from build123d import *

# Parameters (mm, degrees)
SKETCH1_W           = 12
SKETCH1_H           = 75
SKETCH1_W_2         = 50
SKETCH1_H_2         = 12
BOSS_EXTRUDE1_DEPTH = 12


with BuildPart() as part:
    # Sketch1 → Boss-Extrude1 (new body)
    with BuildSketch(Plane(origin=(0, 0, 0), x_dir=(1, 0, 0), z_dir=(0, 1, 0))):
        with Locations((-6, 75)):
            Rectangle(SKETCH1_W, SKETCH1_H)
        Polygon((0, 37.5), (0, 0), (25, 0), (25, 12), (75, 12), (75, 0), (100, 0), (0, 150), (0, 112.5), (12, 112.5), (12, 37.5), align=None)
        with Locations((50, -6)):
            Rectangle(SKETCH1_W_2, SKETCH1_H_2)
        with Locations((50, 6)):
            Rectangle(SKETCH1_W_2, SKETCH1_H_2)
        with Locations((6, 75)):
            Rectangle(SKETCH1_W, SKETCH1_H)
    extrude(amount=BOSS_EXTRUDE1_DEPTH)


solid = part.part
Geometry check sheet. Reference: the model listing, model coordinates, mm. A direction names the side the tool comes from. Give positions to 0.01 mm unless a question says otherwise; leave off trailing zeros. Loops run counter-clockwise (first coordinate to the right, second up) from the corner with the lowest first, then second, coordinate; pieces in that order, holes last. Notation, with made-up numbers: (64.25, 45) -> (100.25, 45) arc R22 cw to (100.25, 82) -> close; hole circle Ø8 at (-35.5, 77.5). An arc over 180 degrees is marked (long way). Answer in a Markdown table with one row per item. Add a question column.
1) Set-up check for faces 1 (the face through (25, 6, 6)), 2 (the face through (50.7, 5.92, -73.95)), 3 (the face through (-12, 6, -74)), 4 (the face through (75, 6, 6)), 5 (the face through (0, 6, -132)): record each of +Z, -Z, +X, -X, +Y, -Y from which the full face is reachable in a straight line by a thin tool's end or side.
2) Cross-section at B-B on z = -130.5. Record the boundary of the cut face in (x, y).
3) Cross-section at C-C on x = 9.5. Record the boundary of the cut face in (y, z), and give its area (3 significant figures).
4) Cross-section at A-A on y = 9.5. Record the boundary of the cut face in (x, z), and give its area (3 significant figures).
5) Material ranges on probe 1 along X at (y, z) = (6.5, -21.5); probe 2 along Z at (x, y) = (24, 1.75); probe 3 along Z at (x, y) = (30, 5.75), recorded low to high. Write a range as from..to.
6) Gauge pin test, flat ends, axial feed: P1, Ø3.5, axis at y = 8, z = -24, coming from the -X side; P2, Ø3, axis at x = 68.5, y = 9.5, coming from the -Z side; P3, Ø6, axis at x = -8, y = 7.5, coming from the +Z side. Record the tip position at first contact, or that the pin passes through.
Outcome:
| question | item | result |
|---|---|---|
| 1 | face 1 | +Z, -X, +Y, -Y |
| 1 | face 2 | -Z, +X, +Y, -Y |
| 1 | face 3 | +Z, -Z, -X, +Y, -Y |
| 1 | face 4 | +Z, +X, +Y, -Y |
| 1 | face 5 | -Z, -X, +Y, -Y |
| 2 | outline | (0, 0) -> (13, 0) -> (13, 12) -> (0, 12) -> close |
| 3 | outline | (0, -135.75) -> (12, -135.75) -> (12, 0) -> (0, 0) -> close |
| 3 | area | 1,630 mm^2 |
| 4 | outline | (-12, -112.5) -> (0, -112.5) -> (0, -150) -> (100, 0) -> (75, 0) -> (75, 12) -> (25, 12) -> (25, 0) -> (0, 0) -> (0, -37.5) -> (-12, -37.5) -> close |
| 4 | area | 9,000 mm^2 |
| 5 | probe 1 | x = 0..85.67 |
| 5 | probe 2 | z = -114..0 |
| 5 | probe 3 | z = -105..12 |
| 6 | P1 | stops at x = 0 |
| 6 | P2 | stops at z = -49.5 |
| 6 | P3 | stops at z = -37.5 |
